For this review, take the finished solid that the model builds, in its own axes (mm). Coordinates: 2 decimals unless noted, no trailing zeros. Order: outer loops, then holes, each group sorted by start corner. A loop starts at its lowest first (then second) coordinate and runs counter-clockwise, first axis right, second up. Notation, with made-up numbers: (34, -3.75) -> (92, -3.75) arc R16 ccw to (92, 13.25) -> close; hole circle Ø10 at (-19.75, 48.25). An arc over 180 degrees is marked (long way). Return JSON: item names as keys, results as strings. Group by question number.
Item 1: For line 1 along Z through (x, y) = (-32, 0); line 2 along Y through (x, z) = (-21, 0); line 3 along Z through (x, y) = (5, 68), list the stretches that pass through material, from the lowest coordinate up.
Item 2: Take a section at B-B (x = 0). Write out the cut boundary in (y, z).
Item 3: Insertion check: pin 1 (4 mm diameter, centred on x = 4.5, y = 8, fed in from +Z); pin 2 (2 mm diameter, centred on x = 36.5, y = 47.5, fed in from -Z); pin 3 (10 mm diameter, centred on x = -41, y = 29, fed in from +Z). Each pin has a flat end and moves straight along its axis. Give the tip position at first contact, or say it passes through.
Item 4: Take a section at C-C (z = -27.5). Count the separate pieces of the cut face and the enclosed holes in it, then the cut area to 3 significant figures.
Item 5: Take a section at D-D (y = 89). Write out the cut boundary in (x, z).
Item 6: Take a section at A-A (y = 30). Write out the cut boundary in (x, z), then the cut area to 3 significant figures.
Item 7: Draft analysis for pull direction X (two halves, no side actions). For faces 1 (the flat face through (-60, 38, -47)), 2 (the cylindrical face through (-36.509, 73.457, 47.614)), 3 (the cylindrical face through (23.923, 82.743, -37.523)), state which applies: +X half, -X half, draft (parallel to the pull), parting line (faces both ways), or undercut.
```python
from build123d import *
from build123d.topology import SkipClean

# Parameters (mm, degrees)
SKETCH1_W                  = 120
SKETCH1_H                  = 63.5
SKETCH2_W                  = 60
SKETCH2_H                  = 88.209377114
HOLE1_D                    = 120
M80_CLEARANCE_HOLE1_REACH  = 195.361
M80_CLEARANCE_HOLE1_BORE_R = 44.5
FILLET1_R                  = 3


with BuildPart() as part:
    # Sketch1 → Revolve1 (revolve)
    with BuildSketch(Plane(origin=(0, 0, 0), x_dir=(-1, 0, 0), z_dir=(0, 0, -1)), mode=Mode.PRIVATE) as revolve1_sk:
        with Locations((0, 31.75)):
            Rectangle(SKETCH1_W, SKETCH1_H)
    revolve(revolve1_sk.sketch.rotate(Axis((60, 0, 0), (-1, 0, 0)), 270), axis=Axis((60, 0, 0), (-1, 0, 0)))

    # Sketch2 → Revolve2 (revolve)
    with SkipClean():  # the faces are left unmerged after this step: merging them gives an invalid solid
        with BuildSketch(Plane.XY, mode=Mode.PRIVATE) as revolve2_sk:
            with Locations((30, 64.895311443)):
                Rectangle(SKETCH2_W, SKETCH2_H)
        revolve(revolve2_sk.sketch.rotate(Axis((0, 109, 0), (0, -1, 0)), 270), axis=Axis((0, 109, 0), (0, -1, 0)))

    # Hole1 (through all)
    with Locations(Plane.ZY.offset(60)):
        with Locations((0, 0)):
            Hole(HOLE1_D / 2)

    # M80 Clearance Hole1 bore → M80 Clearance Hole1 (cut, up to next)
    with BuildSketch(Plane(origin=(0, 109, 0), x_dir=(1, 0, 0), z_dir=(0, 1, 0)), mode=Mode.PRIVATE) as m80_clearance_hole1_sk1:
        Circle(M80_CLEARANCE_HOLE1_BORE_R)
    m80_clearance_hole1_tool1 = extrude(m80_clearance_hole1_sk1.sketch, amount=-M80_CLEARANCE_HOLE1_REACH, mode=Mode.PRIVATE) & part.part
    add(m80_clearance_hole1_tool1.solids().sort_by_distance((0, 109, 0))[0], mode=Mode.SUBTRACT)

    # Fillet1
    fillet1_edges = [part.edges().sort_by_distance(p)[0] for p in [
        (0, 109, 60),
    ]]
    fillet(fillet1_edges, radius=FILLET1_R)


solid = part.part
```
Findings below:
{
 "1": {"line 1": "z = -63.5 to -60, 60 to 63.5", "line 2": "y = -63.5 to -60", "line 3": "z = -59.79 to -44.22, 44.22 to 59.79"},
 "2": {"outline": "(20.79, -60) -> (106, -60) arc R3 ccw to (109, -57) -> (109, -44.5) -> (40.25, -44.5) arc R60 cw (long way) to (40.25, 44.5) -> (109, 44.5) -> (109, 57) arc R3 ccw to (106, 60) -> (20.79, 60) arc R63.5 ccw (long way) to start"},
 "3": {"pin 1": "stops at z = 63.22", "pin 2": "stops at z = -48.37", "pin 3": "stops at z = 58.79"},
 "4": {"separate pieces": "3", "enclosed holes": "0", "area": "2,560 mm2"},
 "5": {"outline": "circle Ø120 at (0, 0); hole circle Ø89 at (0, 0)"},
 "6": {"outline": "(-60, -55.97) -> (-21.63, -55.97) arc R60 ccw to (21.63, -55.97) -> (60, -55.97) -> (60, -51.96) -> (-60, -51.96) -> close; (-60, 51.96) -> (60, 51.96) -> (60, 55.97) -> (21.63, 55.97) arc R60 ccw to (-21.63, 55.97) -> (-60, 55.97) -> close", "area": "1,200 mm2"},
 "7": {"face 1": "-X half", "face 2": "parting line", "face 3": "undercut"}
}
